For this review, take the finished solid that the model builds, in its own axes (mm). Face numbers are marked on the shaded views. Give positions to 0.01 mm unless a question says otherwise; leave off trailing zeros. Order: outer loops, then holes, each group sorted by start corner. A loop starts at its lowest first (then second) coordinate and runs counter-clockwise, first axis right, second up. Notation, with made-up numbers: (52, 0.25) - (108, 0.25) arc R26 cw to (108, 28.25) - close; hole circle Ø6 at (13, 33.25). An arc over 180 degrees is marked (long way). Put each result on its own line as item: value. Start each with the question number.
```python
from build123d import *

# Parameters (mm, degrees)
BOSS_EXTRUDE1_DEPTH = 20
FILLET1_R           = 10
SKETCH2_R           = 2.5000000000000018
CUT_EXTRUDE1_DEPTH  = 37.40054944640259
FILLET2_R           = 0.5


with BuildPart() as part:
    # Sketch1 → Boss-Extrude1 (new body)
    with BuildSketch(Plane(origin=(0, 0, 0), x_dir=(1, 0, 0), z_dir=(0, 1, 0))):
        with BuildLine():
            Line((-15.875000000000004, 0), (-15.875, 30))
            Line((-15.875, 30), (-10.875, 30))
            Line((-10.875, 30), (-10.874999999999996, 11.565033506220383))
            ThreePointArc((-10.874999999999996, 11.565033506220383), (-14.57148328070962, 6.299801584177079), (-15.875000000000004, 0))
        make_face()
    extrude(amount=BOSS_EXTRUDE1_DEPTH)

    # Fillet1
    fillet1_edges = [part.edges().sort_by_distance(p)[0] for p in [
        (-13.375, 0, -30),
        (-13.375, 20, -30),
    ]]
    fillet(fillet1_edges, radius=FILLET1_R - 0.0001)  # a hair under: the kernel refuses the full size

    # Sketch2 → Cut-Extrude1 (cut, through all)
    with BuildSketch(Plane.ZY.offset(15.875000000000004)):
        with Locations((-19.999999999999996, 10)):
            Circle(SKETCH2_R)
    extrude(amount=-CUT_EXTRUDE1_DEPTH, mode=Mode.SUBTRACT)

    # Fillet2
    fillet2_edges = [part.edges().sort_by_distance(p)[0] for p in [
        (-15.875000000000004, 10, 2.2e-16),
    ]]
    fillet(fillet2_edges, radius=FILLET2_R)


solid = part.part
```
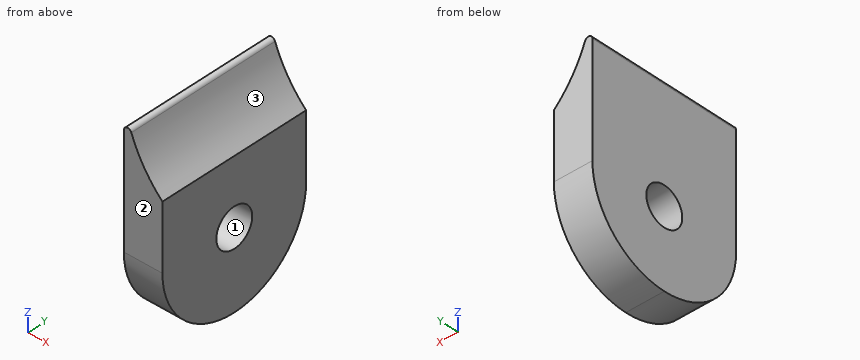
1. Wall thickness on line 1 (Y direction, x = -11.9, z = -20); line 2 (Y direction, x = -13.15, z = -19.5); line 3 (Y direction, x = -15.55, z = -27.5): over which ranges is each line inside the solid? List them lowest first. Write a range as from..to.
2. Add section D-D, the plane y = 16. Give the boundary of the cut face in (x, z) (3 decimals), then the cut area to 3 significant figures.
3. Add section A-A, the plane z = -18. Give the boundary of the cut face in (x, y) (3 decimals), then the cut area to 3 significant figures.
4. The part is to be moulded in two halves that separate along Z. For the marked faces 1, 2 and 3, say which applies: released by +Z, released by -Z, zero draft, split by the parting line, or undercut.
5. Add section B-B, the plane y = 10.75. Give the boundary of the cut face in (x, z) (3 decimals).
6. Clearance check with flat-ended pins moving along their axes: pin 1 (1.5 mm diameter, centred on x = -15, y = 11.5, fed in from +Z); pin 2 (4 mm diameter, centred on y = 10, z = -20, fed in from -X). State where each tip first meets the part, or that it passes through.
Found:
1. line 1: y = 0..7.5, 12.5..20
1. line 2: y = 0..7.55, 12.45..20
1. line 3: y = 3.39..16.61
2. outline: (-15.875, -28) - (-10.875, -28) - (-10.875, -11.565) arc R15.875 cw to (-14.906, -5.463) arc R0.5 ccw to (-15.875, -5.635) - close
2. area: 98.5 mm^2
3. outline: (-15.875, 0) - (-10.875, 0) - (-10.875, 8.5) - (-15.875, 8.5) - close; (-15.875, 11.5) - (-10.875, 11.5) - (-10.875, 20) - (-15.875, 20) - close
3. area: 85.0 mm^2
4. face 1: undercut
4. face 2: zero draft
4. face 3: released by +Z
5. outline: (-15.875, -29.972) - (-10.875, -29.972) - (-10.875, -22.385) - (-15.875, -22.385) - close; (-15.875, -17.615) - (-10.875, -17.615) - (-10.875, -11.565) arc R15.875 cw to (-14.906, -5.463) arc R0.5 ccw to (-15.875, -5.635) - close
6. pin 1: stops at z = -5.13
6. pin 2: passes through
